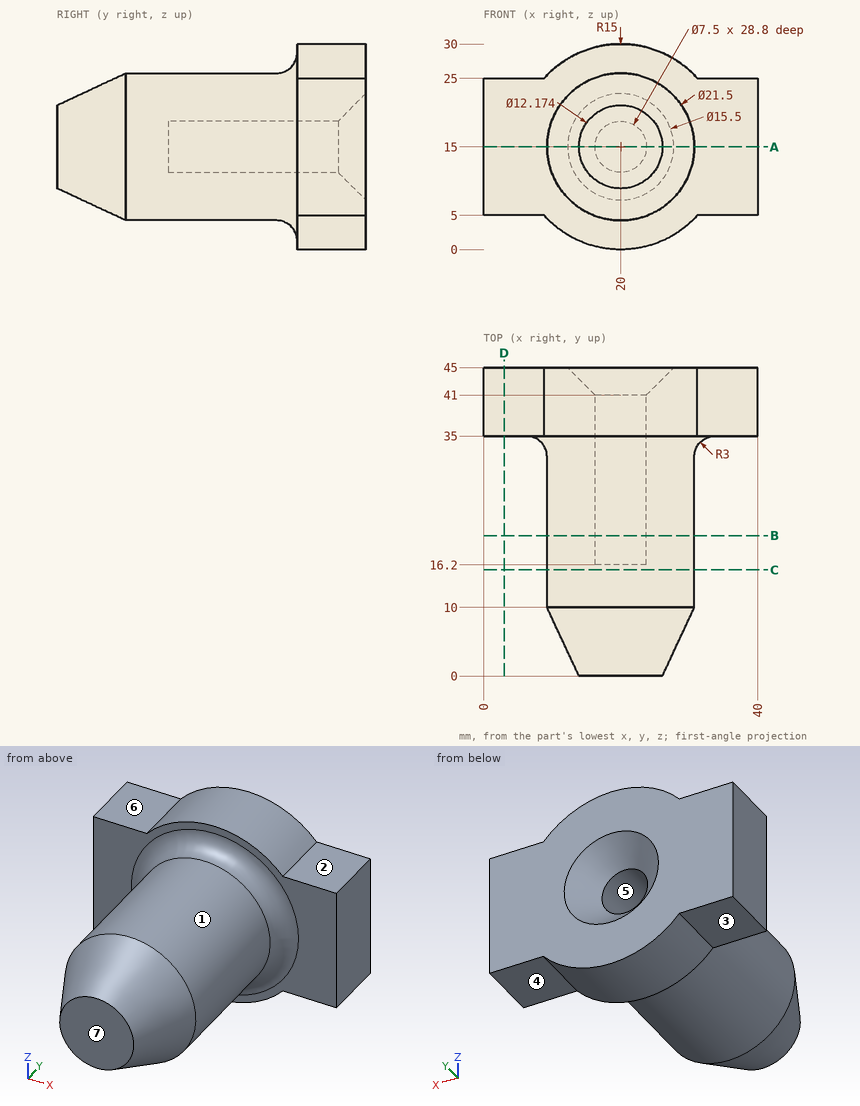
Could you check a few things on this drawing? It's one solid part, dimensions in mm from its lowest x, y, z. A direction names the side the tool comes from. Coordinates: 2 decimals unless noted, no trailing zeros. Order: outer loops, then holes, each group sorted by start corner. A loop starts at its lowest first (then second) coordinate and runs counter-clockwise, first axis right, second up. Notation, with made-up numbers: (-19.5, 77) - (29.5, 77) arc R9 cw to (29.5, 88) - close; hole circle Ø5 at (13.25, 85.25). An arc over 180 degrees is marked (long way). One line per question, with ' | ' between items.
(1) Suppose I cut it at C-C on y = 15.5. List the corners of the cut face in (x, z) for me.
Report:
outline: circle Ø21.5 at (20, 15)
(2) If we mould it in two halves opening along Z, with no side actions, what happens to the marked faces 5, 6 and 7? For each: pulls with the +Z half, pulls with the -Z half, needs draft (parallel to the pull), parting line crosses it, or undercut.
Report:
face 5: undercut | face 6: pulls with the +Z half | face 7: needs draft
(3) Suppose I cut it at A-A on z = 15. List the corners of the cut face in (x, y) for me, and give its area (3 significant figures).
Report:
outline: (0, 35) - (6.25, 35) arc R3 cw to (9.25, 32) - (9.25, 10) - (13.91, 0) - (26.09, 0) - (30.75, 10) - (30.75, 32) arc R3 cw to (33.75, 35) - (40, 35) - (40, 45) - (27.75, 45) - (23.75, 41) - (23.75, 16.2) - (16.25, 16.2) - (16.25, 41) - (12.25, 45) - (0, 45) - close | area: 878 mm2
(4) If I drill on L1, parallel to X at y = 25.5, z = 15; L2, parallel to Y at x = 28, z = 26.5; L3, parallel to Y at x = 29, z = 15, over which ranges is the centre line in solid material (lowest first)?
Report:
L1: x = 9.25 to 16.25, 23.75 to 30.75 | L2: y = 35 to 45 | L3: y = 6.25 to 45
(5) Suppose I cut it at B-B on y = 20.5. List the corners of the cut face in (x, z) for me, and give its area (3 significant figures).
Report:
outline: circle Ø21.5 at (20, 15); hole circle Ø7.5 at (20, 15) | area: 319 mm2
(6) For the marked faces 1, 2, 3 and 4, which set-ups out of +Z, -Z, +X, -X, +Y, -Y let a thin tool reach every point of the face, with its end or its side?
Report:
face 1: -Y | face 2: +Z, +X, +Y, -Y | face 3: -Z, -X, +Y, -Y | face 4: -Z, +X, +Y, -Y
(7) Suppose I cut it at D-D on x = 3. List the corners of the cut face in (y, z) for me, and give its area (3 significant figures).
Report:
outline: (35, 5) - (45, 5) - (45, 25) - (35, 25) - close | area: 200 mm2
(8) Will these pins go through, and if not, where does the flat tip stop? pin 1 (8 mm diameter, centred on x = 32.5, y = 21.5, fed in from +Z); pin 2 (9.5 mm diameter, centred on x = 34.5, y = 38.5, fed in from +Z); pin 3 (1 mm diameter, centred on x = 28, y = 26, fed in from -Z); pin 4 (10 mm diameter, centred on x = 36, y = 8, fed in from -Z).
Report:
pin 1: stops at z = 21.58 | pin 2: stops at z = 26.4 | pin 3: stops at z = 7.3 | pin 4: passes through
